Input: part model. Units: mm. Frame: model coordinates. A direction names the side the tool comes from. Give positions to 0.01 mm unless a question says otherwise; leave off trailing zeros. Write each loop counter-clockwise with the first axis right and the second up, starting at its lowest first coordinate (ties: lowest second). Pieces come first, ordered by that corner, then holes. Notation, with made-up numbers: (5.5, 44.25) -> (42.5, 44.25) arc R22 ccw to (42.5, 73.25) -> close; hole circle Ø1 at (17.5, 16.5). An arc over 180 degrees is marked (long way). Return JSON: item names as keys, results as strings. Group by question number.
Item 1: Section B-B, the plane y = 1.5. Return loops of the section in (x, z).
Item 2: Line query: line 1 (Y direction, x = 0, z = 2.4); line 2 (X direction, y = 1.5, z = 1.4); line 3 (Y direction, x = -2.5, z = 2.75). Output: solid intervals per line, ascending. Write a range as [from, to].
Item 3: Section D-D, the plane y = 18.5. Return loops of the section in (x, z).
Item 4: Section A-A, the plane x = 0. Return loops of the section in (y, z).
Item 5: Set-up query: faces 5 (the face through (-12.224, 20.946, 1.972)), 6 (the face through (-23.126, 7.233, 1.972)), 7 (the face through (6.15, -24.23, 1.97)). Return all of +Z, -Z, +X, -X, +Y, -Y with unobstructed straight access to the full face (end or side cutting, diameter ignored); none if empty.
Item 6: Mould query, pull axis Y, two halves, no side actions, for faces 1 (the face through (-10.167, -21.187, 1.972)), 2 (the face through (10.226, -21.159, 1.972)), 3 (the face through (12.198, 20.937, 1.972)), 4 (the face through (0, -23.5, 2)). Classes: released by +Y, released by -Y, zero draft, split by the parting line, or undercut.
Item 7: Section C-C, the plane y = -20. Return loops of the section in (x, z).
from build123d import *

# Parameters (mm, degrees)
SKETCH1_R           = 16
BOSS_EXTRUDE1_DEPTH = 4


with BuildPart() as part:
    # Sketch1 → Boss-Extrude1 (new body)
    with BuildSketch(Plane.XY):
        with BuildLine():
            Line((23.658232882, 8.080100055), (22.60887418, 6.410055249))
            ThreePointArc((22.60887418, 6.410055249), (22.910805936, 5.229241948), (23.151110514, 4.034362646))
            Line((23.151110514, 4.034362646), (24.821155321, 2.985003945))
            ThreePointArc((24.821155321, 2.985003945), (24.993754895, -0.558763162), (24.662957214, -4.091276263))
            ThreePointArc((24.662957214, -4.091276263), (22.910805936, -5.229241948), (23.995694883, -7.014743551))
            ThreePointArc((23.995694883, -7.014743551), (22.761033302, -10.340955615), (21.067943537, -13.458891304))
            Line((21.067943537, -13.458891304), (19.107985481, -13.679725541))
            ThreePointArc((19.107985481, -13.679725541), (18.373039838, -14.652010344), (17.588673036, -15.584883087))
            Line((17.588673036, -15.584883087), (17.809507272, -17.544841143))
            ThreePointArc((17.809507272, -17.544841143), (15.146492656, -19.889287575), (12.178413721, -21.833145427))
            ThreePointArc((12.178413721, -21.833145427), (10.196267869, -21.172768396), (9.476723699, -23.13421077))
            ThreePointArc((9.476723699, -23.13421077), (6.106387485, -24.242772776), (2.613063, -24.863063))
            Line((2.613063, -24.863063), (1.218393982, -23.468393982))
            ThreePointArc((1.218393982, -23.468393982), (0, -23.5), (-1.218393982, -23.468393982))
            Line((-1.218393982, -23.468393982), (-2.613063, -24.863063))
            ThreePointArc((-2.613063, -24.863063), (-6.106387485, -24.242772776), (-9.476723699, -23.13421077))
            ThreePointArc((-9.476723699, -23.13421077), (-10.196267869, -21.172768396), (-12.178413721, -21.833145427))
            ThreePointArc((-12.178413721, -21.833145427), (-15.146492656, -19.889287575), (-17.809507272, -17.544841143))
            Line((-17.809507272, -17.544841143), (-17.588673036, -15.584883087))
            ThreePointArc((-17.588673036, -15.584883087), (-18.373039838, -14.652010344), (-19.107985481, -13.679725541))
            Line((-19.107985481, -13.679725541), (-21.067943537, -13.458891304))
            ThreePointArc((-21.067943537, -13.458891304), (-22.761033302, -10.340955615), (-23.995694883, -7.014743551))
            ThreePointArc((-23.995694883, -7.014743551), (-22.910805936, -5.229241948), (-24.662957214, -4.091276263))
            ThreePointArc((-24.662957214, -4.091276263), (-24.993754895, -0.558763162), (-24.821155321, 2.985003945))
            Line((-24.821155321, 2.985003945), (-23.151110514, 4.034362646))
            ThreePointArc((-23.151110514, 4.034362646), (-22.910805936, 5.229241948), (-22.60887418, 6.410055249))
            Line((-22.60887418, 6.410055249), (-23.658232882, 8.080100055))
            ThreePointArc((-23.658232882, 8.080100055), (-22.276156802, 11.347812041), (-20.445418397, 14.386968637))
            ThreePointArc((-20.445418397, 14.386968637), (-18.373039838, 14.652010344), (-18.575790893, 16.731407374))
            ThreePointArc((-18.575790893, 16.731407374), (-16.020209918, 19.192521309), (-13.141967154, 21.267080179))
            Line((-13.141967154, 21.267080179), (-11.280289579, 20.615651021))
            ThreePointArc((-11.280289579, 20.615651021), (-10.196267869, 21.172768396), (-9.084819485, 21.672933694))
            Line((-9.084819485, 21.672933694), (-8.433390327, 23.534611269))
            ThreePointArc((-8.433390327, 23.534611269), (-5.01687988, 24.491445778), (-1.499324848, 24.955))
            ThreePointArc((-1.499324848, 24.955), (0, 23.5), (1.499324848, 24.955))
            ThreePointArc((1.499324848, 24.955), (5.01687988, 24.491445778), (8.433390327, 23.534611269))
            Line((8.433390327, 23.534611269), (9.084819485, 21.672933694))
            ThreePointArc((9.084819485, 21.672933694), (10.196267869, 21.172768396), (11.280289579, 20.615651021))
            Line((11.280289579, 20.615651021), (13.141967154, 21.267080179))
            ThreePointArc((13.141967154, 21.267080179), (16.020209918, 19.192521309), (18.575790893, 16.731407374))
            ThreePointArc((18.575790893, 16.731407374), (18.373039838, 14.652010344), (20.445418397, 14.386968637))
            ThreePointArc((20.445418397, 14.386968637), (22.276156802, 11.347812041), (23.658232882, 8.080100055))
        make_face()
        Circle(SKETCH1_R, mode=Mode.SUBTRACT)
    extrude(amount=BOSS_EXTRUDE1_DEPTH)


solid = part.part
Answer below:
{
 "1": {"outline": "(-24.95, 0) -> (-15.93, 0) -> (-15.93, 4) -> (-24.95, 4) -> close; (15.93, 0) -> (24.95, 0) -> (24.95, 4) -> (15.93, 4) -> close"},
 "2": {"line 1": "y = [-23.5, -16], [16, 23.5]", "line 2": "x = [-24.95, -15.93], [15.93, 24.95]", "line 3": "y = [-24.75, -15.8], [15.8, 24.87]"},
 "3": {"outline": "(-16.82, 0) -> (16.82, 0) -> (16.82, 4) -> (-16.82, 4) -> close"},
 "4": {"outline": "(-23.5, 0) -> (-16, 0) -> (-16, 4) -> (-23.5, 4) -> close; (16, 0) -> (23.5, 0) -> (23.5, 4) -> (16, 4) -> close"},
 "5": {"face 5": "+Z, -Z, +Y", "face 6": "+Z, -Z, -X", "face 7": "+Z, -Z, +X, -Y"},
 "6": {"face 1": "undercut", "face 2": "undercut", "face 3": "released by +Y", "face 4": "released by -Y"},
 "7": {"outline": "(-15, 0) -> (15, 0) -> (15, 4) -> (-15, 4) -> close"}
}
